CAD build for the part. Positions are in the model's coordinates, mm. A direction names the side the tool comes from. Coordinates: 2 decimals unless noted, no trailing zeros. Loops run counter-clockwise (first coordinate to the right, second up) from the corner with the lowest first, then second, coordinate; pieces in that order, holes last. Notation, with made-up numbers: (-29, 54) -> (27, 54) arc R12 cw to (27, 59) -> close; hole circle Ø3 at (-36.5, 25.5). An arc over 180 degrees is marked (long way). Return JSON: item names as keys, results as strings. Group by question number.
(1) Saw through at C-C on x = 114.5. Write the cut outline in (y, z).
(2) Tool access for faces 1 (the face through (-22.857, -8, -30)), 2 (the face through (240.143, -6, -30)), 3 (the face through (-73, 0, -30)), 4 (the face through (289, 0, -30)): list every direction of +Z, -Z, +X, -X, +Y, -Y with a clear straight run to the whole face (end or side of a thin tool).
(3) Flat gauge pins, fed straight in: pin 1 Ø10 at (x, z) = (-76, -38.5) entering from -Y; pin 2 Ø10 at (y, z) = (-11.5, -43.5) entering from +X; pin 3 Ø1.5 at (y, z) = (-3, -32.5) entering from -X; pin 4 Ø15 at (x, z) = (107.64, -30) entering from -Y. Where does each tip first touch, or does it go through?
(4) Saw through at D-D on z = -12.5. Write the cut outline in (x, y).
(5) Saw through at A-A on y = -9. Write the cut outline in (x, z).
(6) Saw through at B-B on z = -30. Write the cut outline in (x, y).
(7) Probe L1, parallel to X at y = 1.25, z = -45; L2, parallel to X at y = 0.5, z = -30; L3, parallel to X at y = -6.75, z = -43. List the from-to ranges inside material, lowest first.
```python
from build123d import *

# Parameters (mm, degrees)
BOSS_EXTRUDE1_DEPTH = 60
SKETCH2_R           = 12.5
CUT_EXTRUDE2_DEPTH  = 60


with BuildPart() as part:
    # Sketch1 → Boss-Extrude1 (new body)
    with BuildSketch(Plane.XY):
        Polygon((305.142857143, 0), (272.142857143, 0), (272.142857143, -15.964285714), (238.142857143, -15.964285714), (238.142857143, 0), (-22.857142857, 0), (-22.857142857, -15.964285714), (-56.857142857, -15.964285714), (-56.857142857, 0), (-89.857142857, 0), (-89.857142857, 2), (-54.857142857, 2), (-54.857142857, -13.964285714), (-24.857142857, -13.964285714), (-24.857142857, 2), (240.142857143, 2), (240.142857143, -13.964285714), (270.142857143, -13.964285714), (270.142857143, 2), (305.142857143, 2), align=None)
    extrude(amount=-BOSS_EXTRUDE1_DEPTH)

    # Sketch2 → Cut-Extrude2 (cut)
    with BuildSketch(Plane(origin=(0, 0, 0), x_dir=(1, 0, 0), z_dir=(0, 1, 0))):
        with Locations((107.642857143, 30)):
            Circle(SKETCH2_R)
    extrude(amount=CUT_EXTRUDE2_DEPTH, mode=Mode.SUBTRACT)


solid = part.part
```
Geometry results:
{
 "1": {"outline": "(0, -60) -> (2, -60) -> (2, -40.45) -> (0, -40.45) -> close; (0, -19.55) -> (2, -19.55) -> (2, 0) -> (0, 0) -> close"},
 "2": {"face 1": "+Z, -Z, -Y", "face 2": "+Z, -Z, +Y", "face 3": "+Z, -Z, -X, -Y", "face 4": "+Z, -Z, +X, -Y"},
 "3": {"pin 1": "y = 0", "pin 2": "x = 272.14", "pin 3": "x = -56.86", "pin 4": "through"},
 "4": {"outline": "(-89.86, 0) -> (-56.86, 0) -> (-56.86, -15.96) -> (-22.86, -15.96) -> (-22.86, 0) -> (238.14, 0) -> (238.14, -15.96) -> (272.14, -15.96) -> (272.14, 0) -> (305.14, 0) -> (305.14, 2) -> (270.14, 2) -> (270.14, -13.96) -> (240.14, -13.96) -> (240.14, 2) -> (-24.86, 2) -> (-24.86, -13.96) -> (-54.86, -13.96) -> (-54.86, 2) -> (-89.86, 2) -> close"},
 "5": {"outline": "(-56.86, -60) -> (-54.86, -60) -> (-54.86, 0) -> (-56.86, 0) -> close; (-24.86, -60) -> (-22.86, -60) -> (-22.86, 0) -> (-24.86, 0) -> close; (238.14, -60) -> (240.14, -60) -> (240.14, 0) -> (238.14, 0) -> close; (270.14, -60) -> (272.14, -60) -> (272.14, 0) -> (270.14, 0) -> close"},
 "6": {"outline": "(-89.86, 0) -> (-56.86, 0) -> (-56.86, -15.96) -> (-22.86, -15.96) -> (-22.86, 0) -> (95.14, 0) -> (95.14, 2) -> (-24.86, 2) -> (-24.86, -13.96) -> (-54.86, -13.96) -> (-54.86, 2) -> (-89.86, 2) -> close; (120.14, 0) -> (238.14, 0) -> (238.14, -15.96) -> (272.14, -15.96) -> (272.14, 0) -> (305.14, 0) -> (305.14, 2) -> (270.14, 2) -> (270.14, -13.96) -> (240.14, -13.96) -> (240.14, 2) -> (120.14, 2) -> close"},
 "7": {"L1": "-89.86 to -54.86, -24.86 to 240.14, 270.14 to 305.14", "L2": "-89.86 to -54.86, -24.86 to 95.14, 120.14 to 240.14, 270.14 to 305.14", "L3": "-56.86 to -54.86, -24.86 to -22.86, 238.14 to 240.14, 270.14 to 272.14"}
}
